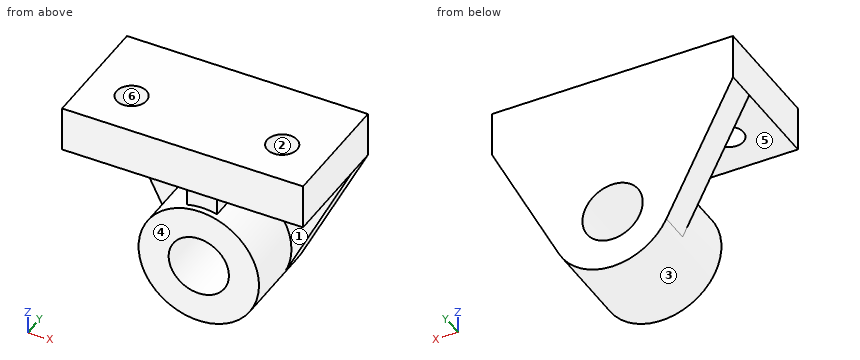
Autodesk Inventor part; units mm, degrees
ref_plane "YZ Plane" through (0, 0, 0) normal (1, 0, 0) x (0, 1, 0)
ref_plane "XZ Plane" through (0, 0, 0) normal (0, 1, 0) x (-1, 0, 0)
ref_plane "XY Plane" through (0, 0, 0) normal (0, 0, 1) x (1, 0, 0)
sketch "Szkic1" plane through (0, 0, 0) normal (0, 0, 1) x (1, 0, 0)
  line L0 (-40, -20) -> (40, -20)
  line L1 (40, -20) -> (40, 20)
  line L2 (40, 20) -> (-40, 20)
  line L3 (-40, 20) -> (-40, -20)
  circle A0 centre (-25, -5) radius 5
  circle A1 centre (25, -5) radius 5
  point P0 (0, 0)
  dimension "d0" = 80
  dimension "d1" = 40
  dimension "d2" = 10
  dimension "d3" = 10
  dimension "d5" = 15
  dimension "d6" = 15
  dimension "d7" = 15
  dimension "d8" = 50
extrude "Wyciągnięcie proste1" add sketch "Szkic1" along normal blind 15
sketch "Szkic3" plane through (-40, 20, 0) normal (0, 1, 0) x (1, 0, 0)
  circle A0 centre (40, 35) radius 20
  circle A1 centre (40, 35) radius 10
  line L0 (80, 0) -> (80, -15)
  line L1 (0, -15) -> (80, -15)
  line L2 (0, 0) -> (22.1342, 43.9895)
  line L3 (80, 0) -> (57.8658, 43.9895)
  line L4 (80, 0) -> (0, 0)
  line L5 (35, 0) -> (35, 15.6351)
  line L6 (45, 0) -> (45, 15.6351)
  point P0 (40, 0)
  dimension "d13" = 40
  dimension "d14" = 20
  dimension "d15" = 40
  dimension "d16" = 50
  dimension "d17" = 10
extrude "Wyciągnięcie proste2" add sketch "Szkic3" against normal blind 30 contours A0
extrude "Wyciągnięcie proste3" add sketch "Szkic3" against normal blind 28 contours L6 L4 L5 A0
extrude "Wyciągnięcie proste4" add sketch "Szkic3" against normal blind 10 contours A0 L3 L4 L6 | A0 L5 L4 L2
properties part number "Bartosz_Zukowski_model_nr_6"
Input: part model. Units: mm. Frame: model coordinates. Face numbers are marked on the shaded views. A direction names the side the tool comes from. Give positions to 0.01 mm unless a question says otherwise; leave off trailing zeros. Write each loop counter-clockwise with the first axis right and the second up, starting at its lowest first coordinate (ties: lowest second). Pieces come first, ordered by that corner, then holes. Notation, with made-up numbers: (3, -35.75) - (12, -35.75) arc R13 cw to (12, -24.75) - close; hole circle Ø10 at (68.5, -16.75). An arc over 180 degrees is marked (long way). Write item = value, one per line. Start each with the question number.
1) Cut plane D-D (x = 25). Return loops of the section in (y, z), and give its area (3 significant figures).
2) Reachability of the marked faces 4, 5 and 6 from +Z, -Z, +X, -X, +Y, -Y: full face, straight path, thin tool, end or side. Return the list, or none.
3) Cut plane B-B (x = 0). Return loops of the section in (y, z).
4) Cut plane A-A (y = -2). Return loops of the section in (x, z).
5) Pin query (flat end, axial travel): pin 1 (4 mm diameter, centred on y = 1.5, z = -4.5, fed in from +X); pin 2 (1 mm diameter, centred on x = 20, y = 10.5, fed in from -Z); pin 3 (5 mm diameter, centred on y = 13.5, z = -9.5, fed in from -X). Return the tip coordinate at first contact, or that it passes through.
6) Draft query along X for the marked faces 1, 2 and 3. Return one class per face: pulls with the +X half, pulls with the -X half, needs draft (parallel to the pull), parting line crosses it, or undercut.
7) Material intervals for L1, parallel to Y at x = 25, z = 8; L2, parallel to X at y = -1.5, z = -35; L3, parallel to Z at x = 0, y = 12, sorted ascending. Write a range as [from, to].
8) Cut plane C-C (z = -35). Return loops of the section in (x, y), and give its area (3 significant figures).
Answers follow:
q1.outline = (-20, 0) - (-10, 0) - (-10, 15) - (-20, 15) - close; (0, 0) - (10, 0) - (10, -29.81) - (20, -29.81) - (20, 15) - (0, 15) - close
q1.area = 748 mm^2
q2.face_4 = -Z, +X, -X, -Y
q2.face_5 = -Y
q2.face_6 = +Z, -Z
q3.outline = (-20, 0) - (-8, 0) - (-8, -15) - (-10, -15) - (-10, -25) - (20, -25) - (20, 15) - (-20, 15) - close; (-10, -55) - (20, -55) - (20, -45) - (-10, -45) - close
q4.outline = (-40, 0) - (-29, 0) - (-29, 15) - (-40, 15) - close; (-21, 0) - (-5, 0) - (-5, -15.64) arc R20 ccw (long way) to (5, -15.64) - (5, 0) - (21, 0) - (21, 15) - (-21, 15) - close; (29, 0) - (40, 0) - (40, 15) - (29, 15) - close; hole circle Ø20 at (0, -35)
q5.pin_1 = 5
q5.pin_2 = -40.74
q5.pin_3 = -36.48
q6.face_1 = needs draft
q6.face_2 = undercut
q6.face_3 = parting line crosses it
q7.L1 = [-20, -10], [0, 20]
q7.L2 = [-20, -10], [10, 20]
q7.L3 = [-55, -45], [-25, 15]
q8.outline = (-22.39, 10) - (-20, 10) - (-20, -10) - (-10, -10) - (-10, 20) - (-22.39, 20) - close; (10, -10) - (20, -10) - (20, 10) - (22.39, 10) - (22.39, 20) - (10, 20) - close
q8.area = 648 mm^2
